Verification items for this drawing (mm, ordinates from the low corner). Round coordinates to 2 decimals unless told otherwise and drop trailing zeros. Order: outer loops, then holes, each group sorted by start corner. A loop starts at its lowest first (then second) coordinate and runs counter-clockwise, first axis right, second up. Notation, with made-up numbers: (-17, -39.5) - (24, -39.5) arc R8 cw to (24, -28.5) - close; hole circle Ø2 at (28.5, 62.25). An arc over 180 degrees is marked (long way). Answer as CSV lines item,"result". Start each with the question number.
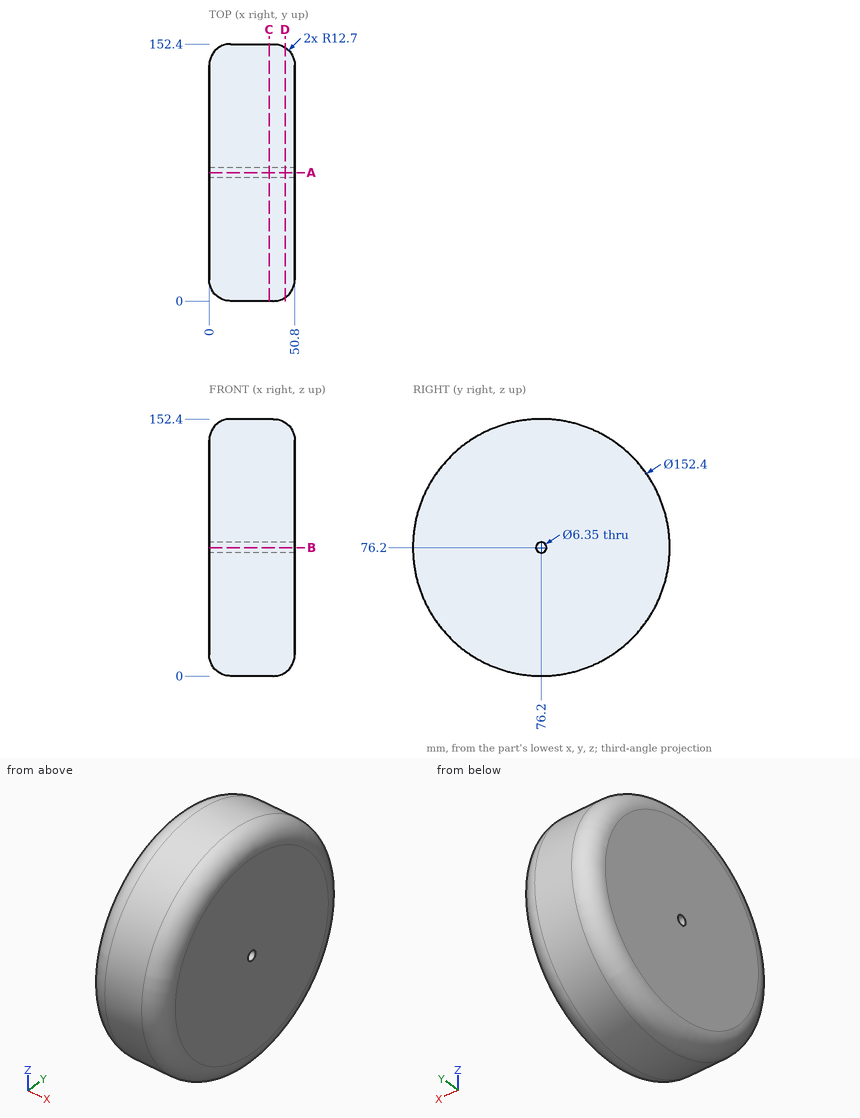
1. Section check C-C on x = 35.5. Record the boundary of the cut face in (y, z) (3 decimals).
2. Thickness scan on probe 1 along Y at (x, z) = (38, 76); probe 2 along Y at (x, z) = (47.5, 75.5). Record the ranges inside material, lowest first.
3. Go/stop test with flat-tipped pins: pin 1 Ø1 at (x, y) = (32, 128.5) entering from -Z; pin 2 Ø4 at (y, z) = (76.2, 76.2) entering from -X; pin 3 Ø3 at (x, y) = (38.5, 55.5) entering from +Z; pin 4 Ø3 at (x, z) = (40.5, 102.5) entering from -Y. Record where each tip stops, or that it passes through.
4. Section check A-A on y = 76.2. Record the boundary of the cut face in (x, z) (3 decimals).
5. Section check D-D on x = 45. Record the boundary of the cut face in (y, z) (3 decimals).
Numbers:
1,outline,"circle Ø152.4 at (76.2, 76.2); hole circle Ø6.35 at (76.2, 76.2)"
2,probe 1,"y = 0 to 73.03, 79.37 to 152.4"
2,probe 2,"y = 4.16 to 73.1, 79.3 to 148.24"
3,pin 1,"stops at z = 20.31"
3,pin 2,"passes through"
3,pin 3,"stops at z = 149.94"
3,pin 4,"stops at y = 4.33"
4,outline,"(0, 12.7) arc R12.7 ccw to (12.7, 0) - (38.1, 0) arc R12.7 ccw to (50.8, 12.7) - (50.8, 73.025) - (0, 73.025) - close; (0, 79.375) - (50.8, 79.375) - (50.8, 139.7) arc R12.7 ccw to (38.1, 152.4) - (12.7, 152.4) arc R12.7 ccw to (0, 139.7) - close"
5,outline,"circle Ø148.324 at (76.2, 76.2); hole circle Ø6.35 at (76.2, 76.2)"
